from build123d import *

# Parameters (mm, degrees)
SKETCH_1_W          = 85
SKETCH_1_H          = 154
EXTRUDE_1_DEPTH     = 3
CUT_EXTRUDE_2_DEPTH = 58
EXTRUDE_2_DEPTH     = 3
SKETCH_4_W          = 44.4
SKETCH_4_H          = 24.3
CUT_EXTRUDE_3_DEPTH = 58


with BuildPart() as part:
    # 草图1 → 凸台-拉伸1 (new body)
    with BuildSketch(Plane.XY):
        with Locations((42.5, -77)):
            Rectangle(SKETCH_1_W, SKETCH_1_H)
    extrude(amount=EXTRUDE_1_DEPTH)

    # 草图2 → 切除-拉伸2 (cut)
    with BuildSketch(Plane.XY.offset(3)):
        Polygon((10.076271632, -27.258966415), (-21.319269453, 4.13657467), (-4.13657467, 21.319269453), (27.258966415, -10.076271632), align=None)
        Polygon((-21.319269453, -158.13657467), (-4.13657467, -175.319269453), (27.258966415, -143.923728368), (10.076271632, -126.741033585), align=None)
        Polygon((74.923728368, -126.741033585), (106.319269453, -158.13657467), (89.13657467, -175.319269453), (57.741033585, -143.923728368), align=None)
        Polygon((74.923728368, -27.258966415), (57.741033585, -10.076271632), (89.13657467, 21.319269453), (106.319269453, 4.13657467), align=None)
        Polygon((85, -41.334617867), (99, -50.011428212), (99, -103.988571788), (85, -112.665382133), align=None)
        Polygon((0, -41.334617867), (-14, -50.011428212), (-14, -103.988571788), (0, -112.665382133), align=None)
    extrude(amount=-CUT_EXTRUDE_2_DEPTH, mode=Mode.SUBTRACT)

    # 草图3 → 凸台-拉伸2 (add)
    with BuildSketch(Plane.XY.offset(3)):
        Polygon((85, -41.334617867), (99, -50.011428212), (99, -103.988571788), (85, -112.665382133), align=None)
        Polygon((-14, -103.988571788), (0, -112.665382133), (0, -41.334617867), (-14, -50.011428212), align=None)
    extrude(amount=-EXTRUDE_2_DEPTH)

    # 草图4 → 切除-拉伸3 (cut)
    with BuildSketch(Plane.XY.offset(3)):
        with Locations((113.2, -77)):
            Rectangle(SKETCH_4_W, SKETCH_4_H)
        with Locations((-28.2, -77)):
            Rectangle(SKETCH_4_W, SKETCH_4_H)
    extrude(amount=-CUT_EXTRUDE_3_DEPTH, mode=Mode.SUBTRACT)


solid = part.part
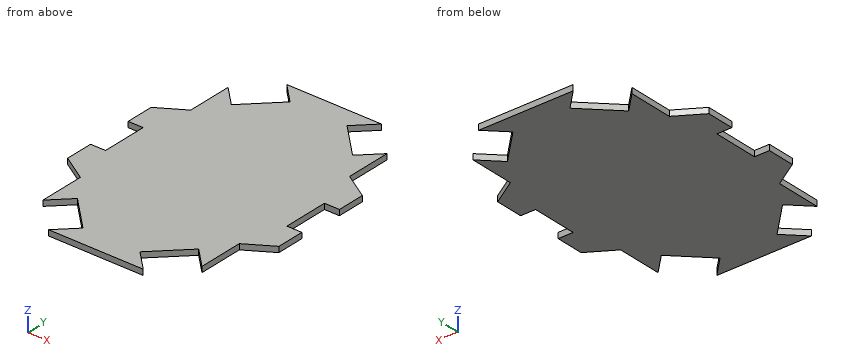
Geometry: final body of the model. Coordinates: model frame, mm. Give positions to 0.01 mm unless a question says otherwise; leave off trailing zeros. Order: outer loops, then holes, each group sorted by start corner. A loop starts at its lowest first (then second) coordinate and runs counter-clockwise, first axis right, second up. Notation, with made-up numbers: (74, 68.25) -> (91, 68.25) arc R26 cw to (91, 103.25) -> close; hole circle Ø2 at (85, -7). An arc over 180 degrees is marked (long way). Answer as a JSON object with one key per item and string values.
Q1. Section D-D (x = 88). Output: boundary loops of the cut face in (y, z), plus the area to 3 significant figures.
Entries:
{"outline": "(-110.81, 0) -> (-43.19, 0) -> (-43.19, 3) -> (-110.81, 3) -> close", "area": "203 mm^2"}
Q2. First-contact query: pin 1 (0.9 mm diameter, centred on x = -10.5, z = 1.5, fed in from +Y); pin 2 (1.5 mm diameter, centred on y = -122, z = 1.5, fed in from -X); pin 3 (1.5 mm diameter, centred on x = 96.5, z = 1.5, fed in from +Y). Flat tips, straight axial feed; report the tip coordinate or a pass-through.
Entries:
{"pin 1": "stops at y = -47.56", "pin 2": "stops at x = 0", "pin 3": "stops at y = -48"}
Q3. Section A-A (x = 63). Output: boundary loops of the cut face in (y, z).
Entries:
{"outline": "(-154, 0) -> (-149.18, 0) -> (-149.18, 3) -> (-154, 3) -> close; (-138.66, 0) -> (-15.34, 0) -> (-15.34, 3) -> (-138.66, 3) -> close; (-4.82, 0) -> (0, 0) -> (0, 3) -> (-4.82, 3) -> close"}
Q4. Material intervals for probe 1 along Y at (x, z) = (61, 2.85); probe 2 along Y at (x, z) = (62, 1.7); probe 3 along X at (y, z) = (-123.5, 2.25), sorted ascending.
Entries:
{"probe 1": "y = -154 to -147.18, -140.66 to -13.34, -6.82 to 0", "probe 2": "y = -154 to -148.18, -139.66 to -14.34, -5.82 to 0", "probe 3": "x = 0 to 85"}
Q5. Section C-C (y = -124.5). Output: boundary loops of the cut face in (x, z).
Entries:
{"outline": "(0, 0) -> (85, 0) -> (85, 3) -> (0, 3) -> close"}
